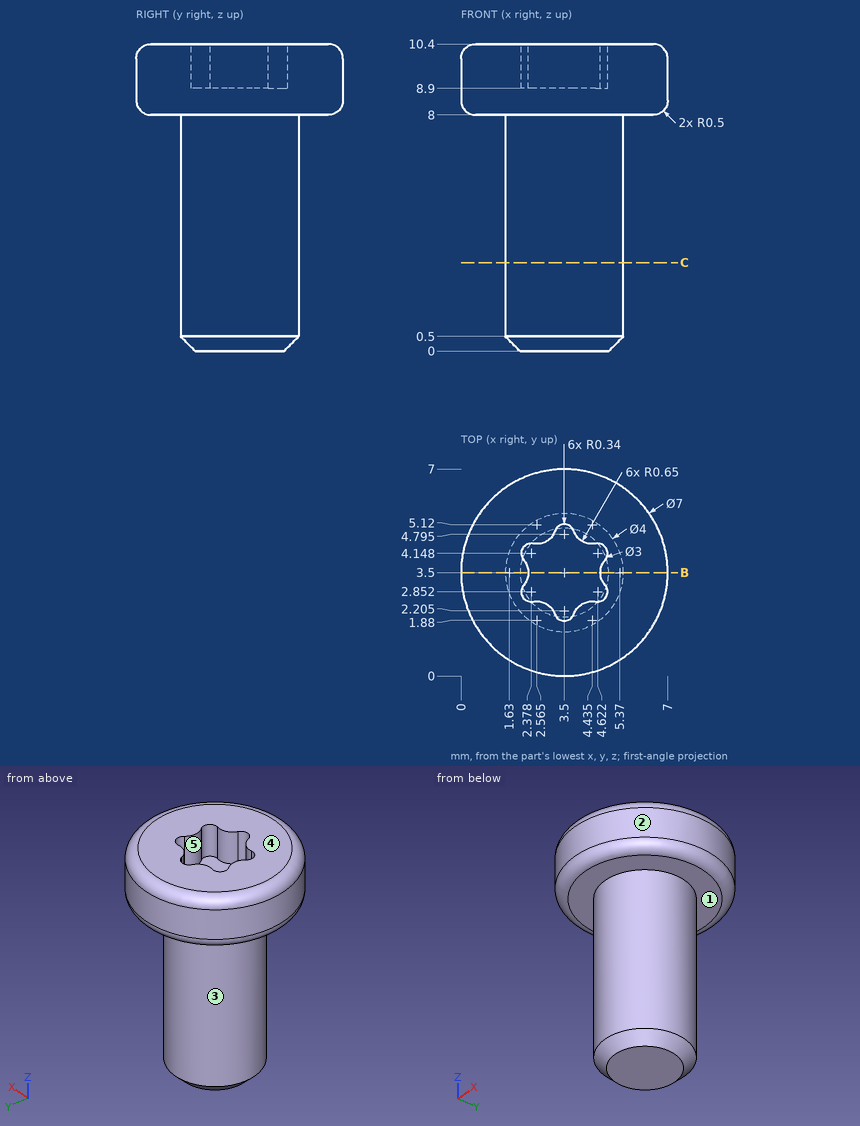
Geometry check sheet. Reference: drawing and pictorial views, mm from the part's lowest x, y, z. A direction names the side the tool comes from. Round coordinates to 2 decimals unless told otherwise and drop trailing zeros. Loops run counter-clockwise (first coordinate to the right, second up) from the corner with the lowest first, then second, coordinate; pieces in that order, holes last.
1. Set-up check for the marked faces 1 and 2: record each of +Z, -Z, +X, -X, +Y, -Y from which the full face is reachable in a straight line by a thin tool's end or side.
2. Scan lines: probe 1 along Z at (x, y) = (5.25, 2); probe 2 along Y at (x, z) = (1.75, 5.5) (1 decimal). Record each from-to range of solid material in increasing order.
3. Mould release check, pull along X, two halves, no side actions. Record for the marked faces 3, 4 and 5: released by +X, released by -X, zero draft, split by the parting line, or undercut.
4. Sectioned sample at B-B on y = 3.5. Record the boundary of the cut face in (x, z).
5. Gauge pin test, flat ends, axial feed: pin 1 Ø2 at (y, z) = (3, 8.5) entering from +X; pin 2 Ø0.9 at (x, y) = (4, 4) entering from +Z; pin 3 Ø4 at (x, z) = (2, 4) entering from -Y; pin 4 Ø1 at (x, y) = (6, 3) entering from -Z. Record the tip position at first contact, or that the pin passes through.
6. Sectioned sample at C-C on z = 3. Record the boundary of the cut face in (x, y).
Recorded:
1. face 1: -Z
1. face 2: +Z, -Z
2. probe 1: z = 8 to 10.4
2. probe 2: y = 2.5 to 4.5
3. face 3: split by the parting line
3. face 4: zero draft
3. face 5: undercut
4. outline: (0, 8.5) arc R0.5 ccw to (0.5, 8) - (1.5, 8) - (1.5, 0.5) - (2, 0) - (5, 0) - (5.5, 0.5) - (5.5, 8) - (6.5, 8) arc R0.5 ccw to (7, 8.5) - (7, 9.9) arc R0.5 ccw to (6.5, 10.4) - (4.72, 10.4) - (4.72, 8.9) - (2.28, 8.9) - (2.28, 10.4) - (0.5, 10.4) arc R0.5 ccw to (0, 9.9) - close
5. pin 1: stops at x = 7
5. pin 2: stops at z = 8.9
5. pin 3: stops at y = 1.5
5. pin 4: stops at z = 8
6. outline: circle Ø4 at (3.5, 3.5)
